```python
from build123d import *

# Parameters (mm, degrees)
BOSS_EXTRUDE1_DEPTH = 5


with BuildPart() as part:
    # Sketch1 → Boss-Extrude1 (new body)
    with BuildSketch(Plane.XY):
        with BuildLine():
            Line((19.615384615, -0.365384615), (19.615384615, -8.365384615))
            Line((19.615384615, -8.365384615), (-20.384615385, -8.365384615))
            Line((-20.384615385, -8.365384615), (-20.384615385, -0.365384615))
            Line((-20.384615385, -0.365384615), (-15.384615385, -0.365384615))
            ThreePointArc((-15.384615385, -0.365384615), (-13.384615385, 1.634615385), (-15.384615385, 3.634615385))
            Line((-15.384615385, 3.634615385), (-20.384615385, 3.634615385))
            Line((-20.384615385, 3.634615385), (-20.384615385, 11.634615385))
            Line((-20.384615385, 11.634615385), (19.615384615, 11.634615385))
            Line((19.615384615, 11.634615385), (19.615384615, 3.634615385))
            Line((19.615384615, 3.634615385), (14.615384615, 3.634615385))
            ThreePointArc((14.615384615, 3.634615385), (12.615384615, 1.634615385), (14.615384615, -0.365384615))
            Line((14.615384615, -0.365384615), (19.615384615, -0.365384615))
        make_face()
    extrude(amount=BOSS_EXTRUDE1_DEPTH)


solid = part.part
```
Can you work these out from the model? Positions are in its coordinate system, mm. A direction names the side the tool comes from. Coordinates: 2 decimals unless noted, no trailing zeros. Loops run counter-clockwise (first coordinate to the right, second up) from the corner with the lowest first, then second, coordinate; pieces in that order, holes last. Notation, with made-up numbers: (87, 57) -> (122, 57) arc R28 cw to (122, 84) -> close; hole circle Ø11 at (24.25, -31.5). An arc over 180 degrees is marked (long way). Put each result on its own line as item: value. Start each with the question number.
Q1. Thinking about a two-plate mould opening in Y: for faces 4 (the face through (0, 2, 5)), 5 (the face through (-1, 11.635, 2)), 6 (the face through (0, -8.365, 2)), 7 (the face through (12.616, 1.679, 2.465)), which applies, pulls with the +Y half, pulls with the -Y half, needs draft (parallel to the pull), parting line crosses it, or undercut?
Q2. I want a section at A-A (x = 16.5). Write out the boundary of the cut face in (y, z).
Q3. I want a section at B-B (z = 3.95). Write out the boundary of the cut face in (x, y).
Q4. If I drill on line 1 (Y direction, x = -16, z = 3); line 2 (Y direction, x = -14, z = 0.65); line 3 (X direction, y = 1.25, z = 0.95), over which ranges is the centre line in solid material (lowest first)? Write a range as [from, to].
Q5. For faces 1 (the face through (17, -0.365, 2)), 2 (the face through (-20.385, 8, 2)), 3 (the face through (-18, -0.365, 2)), which set-ups out of +Z, -Z, +X, -X, +Y, -Y let a thin tool reach every point of the face, with its end or its side?
Taken from the geometry:
1. face 4: needs draft
1. face 5: pulls with the +Y half
1. face 6: pulls with the -Y half
1. face 7: undercut
2. outline: (-8.37, 0) -> (-0.37, 0) -> (-0.37, 5) -> (-8.37, 5) -> close; (3.63, 0) -> (11.63, 0) -> (11.63, 5) -> (3.63, 5) -> close
3. outline: (-20.38, -8.37) -> (19.62, -8.37) -> (19.62, -0.37) -> (14.62, -0.37) arc R2 cw to (14.62, 3.63) -> (19.62, 3.63) -> (19.62, 11.63) -> (-20.38, 11.63) -> (-20.38, 3.63) -> (-15.38, 3.63) arc R2 cw to (-15.38, -0.37) -> (-20.38, -0.37) -> close
4. line 1: y = [-8.37, -0.37], [3.63, 11.63]
4. line 2: y = [-8.37, 0.19], [3.08, 11.63]
4. line 3: x = [-13.42, 12.65]
5. face 1: +Z, -Z, +X
5. face 2: +Z, -Z, -X, +Y, -Y
5. face 3: +Z, -Z, -X
